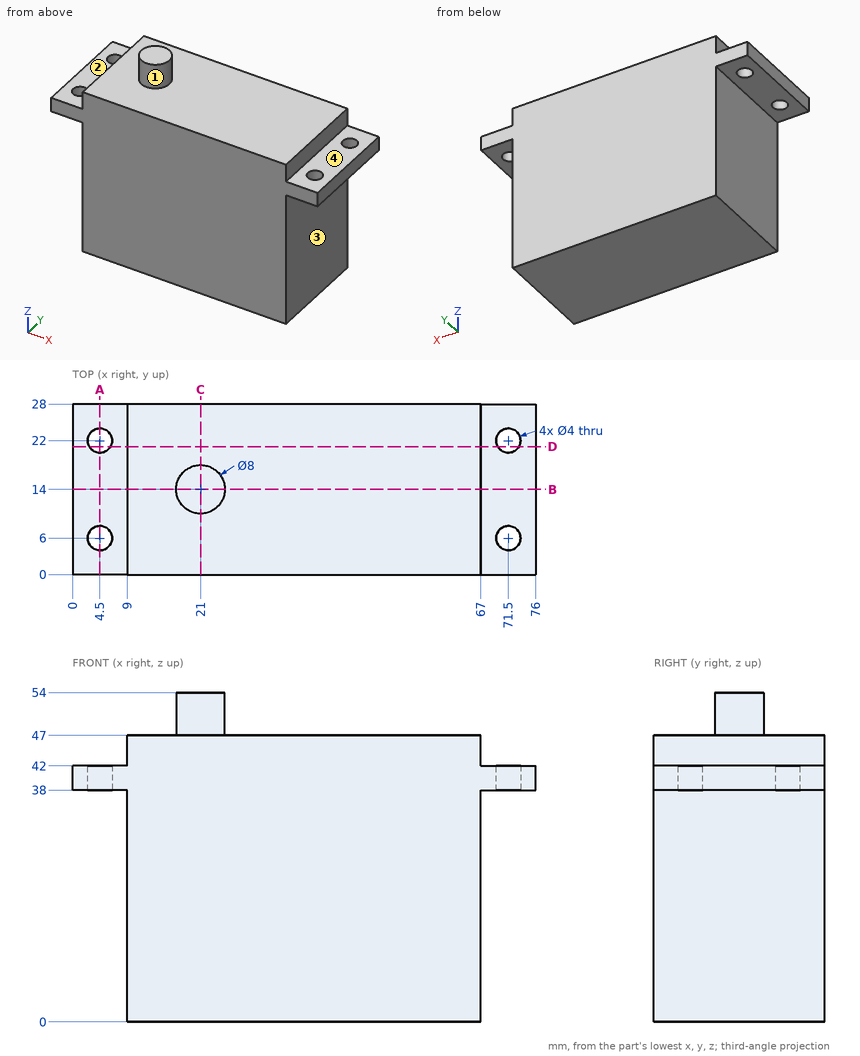
Geometry check sheet. Reference: drawing and pictorial views, mm from the part's lowest x, y, z. A direction names the side the tool comes from. Give positions to 0.01 mm unless a question says otherwise; leave off trailing zeros. Order: outer loops, then holes, each group sorted by start corner. A loop starts at its lowest first (then second) coordinate and runs counter-clockwise, first axis right, second up. Notation, with made-up numbers: (6, -20.75) - (11, -20.75) arc R36 ccw to (11, 14.25) - close; hole circle Ø3 at (-20, 9). An arc over 180 degrees is marked (long way). Answer as CSV lines item,"result".
1. Scan lines: probe 1 along Y at (x, z) = (4.5, 39.65); probe 2 along X at (y, z) = (22, 40.3); probe 3 along Y at (x, z) = (4, 39). Record each from-to range of solid material in increasing order. Write a range as from..to.
Result sheet:
probe 1,"0..4, 8..20, 24..28"
probe 2,"0..2.5, 6.5..69.5, 73.5..76"
probe 3,"0..4.06, 7.94..20.06, 23.94..28"
2. Section check B-B (y = 14). Record the boundary of the cut face in (x, z).
Result sheet:
outline,"(0, 38) - (9, 38) - (9, 0) - (67, 0) - (67, 38) - (76, 38) - (76, 42) - (67, 42) - (67, 47) - (25, 47) - (25, 54) - (17, 54) - (17, 47) - (9, 47) - (9, 42) - (0, 42) - close"
3. Section check A-A (x = 4.5). Record the boundary of the cut face in (y, z).
Result sheet:
outline,"(0, 38) - (4, 38) - (4, 42) - (0, 42) - close; (8, 38) - (20, 38) - (20, 42) - (8, 42) - close; (24, 38) - (28, 38) - (28, 42) - (24, 42) - close"
4. Go/stop test with flat-tipped pins: P1, Ø7, axis at x = 3.5, y = 18, coming from the +Z side; P2, Ø5, axis at y = 21.5, z = 29, coming from the +X side; P3, Ø4, axis at x = 40.5, z = 24.5, coming from the -Y side; P4, Ø2, axis at x = 51, y = 5, coming from the +Z side. Record where each tip stops, or that it passes through.
Result sheet:
P1,"z = 42"
P2,"x = 67"
P3,"y = 0"
P4,"z = 47"
5. Tool access check on the marked faces 1, 2, 3 and 4. Record the directions out of +Z, -Z, +X, -X, +Y, -Y that give a thin tool (end or side, any length) a straight path to the whole face; none if there is none.
Result sheet:
face 1,"+Z"
face 2,"+Z, -X, +Y, -Y"
face 3,"-Z, +X, +Y, -Y"
face 4,"+Z, +X, +Y, -Y"
6. Section check D-D (y = 21). Record the boundary of the cut face in (x, z).
Result sheet:
outline,"(0, 38) - (2.77, 38) - (2.77, 42) - (0, 42) - close; (6.23, 38) - (9, 38) - (9, 0) - (67, 0) - (67, 38) - (69.77, 38) - (69.77, 42) - (67, 42) - (67, 47) - (9, 47) - (9, 42) - (6.23, 42) - close; (73.23, 38) - (76, 38) - (76, 42) - (73.23, 42) - close"
7. Section check C-C (x = 21). Record the boundary of the cut face in (y, z), then the cut area to 3 significant figures.
Result sheet:
outline,"(0, 0) - (28, 0) - (28, 47) - (18, 47) - (18, 54) - (10, 54) - (10, 47) - (0, 47) - close"
area,"1,370 mm²"
